For this review, take the finished solid that the model builds, in its own axes (mm). Face numbers are marked on the shaded views. A direction names the side the tool comes from. Give positions to 0.01 mm unless a question says otherwise; leave off trailing zeros. Order: outer loops, then holes, each group sorted by start corner. A loop starts at its lowest first (then second) coordinate and runs counter-clockwise, first axis right, second up. Notation, with made-up numbers: M 54,89.25 L 102,89.25 A18 cw 102,122.25 Z; hole C 28,76.5 d11. An arc over 180 degrees is marked long. Answer as CSV lines item,"result". Start each with the question number.
1. Machinability: for the marked faces 1, 2 and 3, which of the approach directions +Z, -Z, +X, -X, +Y, -Y give a long, thin tool a straight path to every point of the face, cutting with its end or side? Answer none if there is none.
2. Clearance check with flat-ended pins moving along their axes: P1, Ø1, axis at x = 19, y = 1.5, coming from the -Z side; P2, Ø1.5, axis at y = -1, z = -1.5, coming from the -X side; P3, Ø2, axis at x = -0.5, z = 2, coming from the -Y side. State where each tip first meets the part, or that it passes through.
3. For line 1 along X through (y, z) = (1.2, 0.95); line 2 along Z through (x, y) = (14, -0.2); line 3 along Y through (x, z) = (-21, -1.15), list the stretches that pass through material, from the lowest coordinate up.
4. We need section A-A, the plane z = 0. Give the boundary of the cut face in (x, y), and give its area (3 significant figures).
5. We need section C-C, the plane x = -15. Give the boundary of the cut face in (y, z), and give its area (3 significant figures).
from build123d import *

# Parameters (mm, degrees)
EXTRUDE_1_DEPTH      = 30
EXTRUDE_1_DEPTH_BACK = 30
SKETCH_1_R           = 2.5
SKETCH_2_R           = 1.5
EXTRUDE_2_DEPTH      = 6
EXTRUDE_START        = 6
SKETCH_3_R           = 1.5
EXTRUDE_3_DEPTH      = 6


with BuildPart() as part:
    # Sketch 1 → Extrude 1 (new, two sides: drawn at the far end of the back side and taken through both)
    with BuildSketch(Plane(origin=(0, 0, 0), x_dir=(0, 0, -1), z_dir=(1, 0, 0)).offset(-EXTRUDE_1_DEPTH_BACK)):
        Circle(SKETCH_1_R)
    extrude(amount=EXTRUDE_1_DEPTH + EXTRUDE_1_DEPTH_BACK)

    # Sketch 2 → Extrude 2 (add)
    with BuildSketch(Plane(origin=(30, 0, 0), x_dir=(0, 0, -1), z_dir=(1, 0, 0))):
        Circle(SKETCH_2_R)
    extrude(amount=EXTRUDE_2_DEPTH)

    # Sketch 3 → Extrude 3 (add)
    with BuildSketch(Plane.ZY.offset(30).offset(EXTRUDE_START)):
        with Locations(Location((0, 0, 0), (0, 0, 180))):
            Circle(SKETCH_3_R)
    extrude(amount=-EXTRUDE_3_DEPTH)


solid = part.part
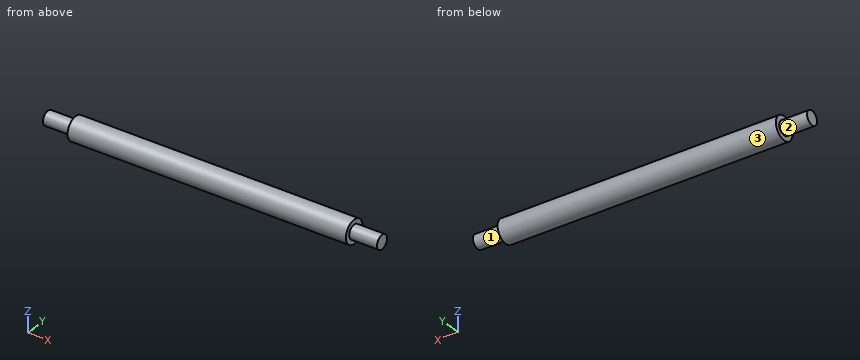
Result set:
1,face 1,"+X"
1,face 2,"-X"
1,face 3,"+X, -X"
2,P1,"z = -2.29"
2,P2,"x = -36"
2,P3,"y = -2.29"
3,line 1,"-30 to 30"
3,line 2,"-2.49 to 2.49"
3,line 3,"-2.22 to 2.22"
4,outline,"M -36,-1.5 L -30,-1.5 L -30,-2.5 L 30,-2.5 L 30,-1.5 L 36,-1.5 L 36,1.5 L 30,1.5 L 30,2.5 L -30,2.5 L -30,1.5 L -36,1.5 Z"
4,area,"336 mm2"
5,outline,"C 0,0 d5"
5,area,"19.6 mm2"
